Part model, mm, in its own coordinate system. A direction names the side the tool comes from. Coordinates: 2 decimals unless noted, no trailing zeros. Write each loop counter-clockwise with the first axis right and the second up, starting at its lowest first coordinate (ties: lowest second). Pieces come first, ordered by that corner, then holes. Notation, with made-up numbers: (61, 89) -> (67, 89) arc R17 cw to (67, 103) -> close; hole circle Ø5 at (88, -7). An arc over 180 degrees is marked (long way). Write item = value, one per line.
from build123d import *

# Parameters (mm, degrees)
EXTRUDE_1_DEPTH     = 25
SKETCH_2_R          = 1.5
CUT_EXTRUDE_1_DEPTH = 8
SKETCH_3_R          = 1.5
CUT_EXTRUDE_2_DEPTH = 8
CUT_EXTRUDE_3_DEPTH = 8
SKETCH_6_R          = 1.5
CUT_EXTRUDE_4_DEPTH = 94.766234905
FILLET_1_R          = 0.5


with BuildPart() as part:
    # 草图1 → 凸台-拉伸1 (new body)
    with BuildSketch(Plane.XY):
        Polygon((0, 0), (-88, 0), (0, 21.94086425), align=None)
    extrude(amount=EXTRUDE_1_DEPTH)

    # 草图2 → 切除-拉伸1 (cut)
    with BuildSketch(Plane.XZ):
        with Locations(Location((-7.5, 19.5, 0), (0, 0, 270))):
            Circle(SKETCH_2_R)
        with Locations(Location((-7.5, 5.5, 0), (0, 0, 90))):
            Circle(SKETCH_2_R)
    extrude(amount=-CUT_EXTRUDE_1_DEPTH, mode=Mode.SUBTRACT)

    # 草图3 → 切除-拉伸2 (cut)
    with BuildSketch(Plane(origin=(-5.150305914, 20.656748763, 0), x_dir=(0.9702957262759981, 0.24192189559966132, 0), z_dir=(-0.2419218955996613, 0.970295726275998, 0))):
        with Locations(Location((-4.692024529, -5.5, 0), (0, 0, 180))):
            Circle(SKETCH_3_R)
        with Locations(Location((-4.692024529, -19.5, 0), (0, 0, 180))):
            Circle(SKETCH_3_R)
    extrude(amount=-CUT_EXTRUDE_2_DEPTH, mode=Mode.SUBTRACT)

    # 草图5 → 切除-拉伸3 (cut)
    with BuildSketch(Plane.XY.offset(22)):
        Polygon((-77.5, 1.371304016), (-77.5, 2.61794403), (-82.5, 1.371304016), align=None)
    cut_extrude_3 = extrude(amount=-CUT_EXTRUDE_3_DEPTH, mode=Mode.SUBTRACT)

    # 草图6 → 切除-拉伸4 (cut, through all)
    with BuildSketch(Plane(origin=(0, 1.371304016, 0), x_dir=(1, 0, 0), z_dir=(0, 1, 0))):
        with Locations(Location((-80.5, -18, 0), (0, 0, 180))):
            Circle(SKETCH_6_R)
    cut_extrude_4 = extrude(amount=-CUT_EXTRUDE_4_DEPTH, mode=Mode.SUBTRACT)

    # 镜向1: 切除-拉伸3, 切除-拉伸4 across plane
    add(cut_extrude_3.mirror(Plane.XY.offset(12.5)), mode=Mode.SUBTRACT)
    add(cut_extrude_4.mirror(Plane.XY.offset(12.5)), mode=Mode.SUBTRACT)

    # 圆角1
    fillet_1_edges = [part.edges().sort_by_distance(p)[0] for p in [
        (-80, 1.371304016, 14),
        (-77.5, 1.371304016, 18),
        (-77.5, 1.994624023, 14),
        (-80, 1.371304016, 22),
        (-77.5, 1.994624023, 22),
        (-80, 1.371304016, 3),
        (-77.5, 1.994624023, 3),
        (-77.5, 1.371304016, 7),
        (-80, 1.371304016, 11),
        (-77.5, 1.994624023, 11),
    ]]
    fillet(fillet_1_edges, radius=FILLET_1_R)


solid = part.part
Q1. Saw through at C-C on z = 2. Give the cut face in (x, y), and give its area (3 significant figures).
Model answer:
outline = (-88, 0) -> (0, 0) -> (0, 21.94) -> close
area = 965 mm²
Q2. Mould opens along Y. For faces 6 (the face through (-43, 0, 12)), 7 (the face through (-7.59, 15.98, 4.59)), 8 (the face through (-24, 6, 0)) say: released by +Y, released by -Y, zero draft, split by the parting line, or undercut.
Model answer:
face_6 = released by -Y
face_7 = undercut
face_8 = zero draft
Q3. Saw through at D-D on x = -65.5. Give the cut face in (y, z), and give its area (3 significant figures).
Model answer:
outline = (0, 0) -> (5.61, 0) -> (5.61, 25) -> (0, 25) -> close
area = 140 mm²
Q4. Pin check, flat tips, straight feed: pin 1 (3 mm diameter, centred on x = -63.5, z = 20.5, fed in from +Y); pin 2 (0.5 mm diameter, centred on x = -79.5, y = 2.5, fed in from +Z) (3 decimals); pin 3 (1.8 mm diameter, centred on x = -7.5, z = 5.5, fed in from +Y); pin 4 (4 mm diameter, centred on x = -80.5, z = 7, fed in from +Y). Stop position of each tip, or through.
Model answer:
pin_1 = 6.48
pin_2 = through
pin_3 = 20.3
pin_4 = 1.37
Q5. Probe line 1 (Z direction, x = -80.5, y = 0.35); line 2 (X direction, y = 2.5, z = 5.5); line 3 (Z direction, x = -8.5, y = 18.5). List the from-to ranges inside material, lowest first. Write a range as from..to.
Model answer:
line_1 = 0..5.5, 8.5..16.5, 19.5..25
line_2 = -77.5..-9, -6..0
line_3 = 0..4.32, 6.68..18.32, 20.68..25
Q6. Saw through at B-B on x = -7.5. Count the separate pieces of the cut face and the enclosed holes in it, and give its area (3 significant figures).
Model answer:
separate_pieces = 1
enclosed_holes = 2
area = 431 mm²
Q7. Saw through at A-A on y = 6.5. Give the cut face in (x, z), and give its area (3 significant figures).
Model answer:
outline = (-61.93, 0) -> (0, 0) -> (0, 25) -> (-61.93, 25) -> close; hole circle Ø3 at (-7.5, 5.5); hole circle Ø3 at (-7.5, 19.5)
area = 1,530 mm²
Q8. Which spindle directions (+Z, -Z, +X, -X, +Y, -Y) get a long thin tool onto all of the face, cutting with end or side? Do faces 1 (the face through (-24, 6, 25)), 2 (the face through (-8.4, 3.9, 20.7)), 3 (the face through (-78.8, 1.371, 7)), 4 (the face through (-81.886, 0.695, 7.575)), 5 (the face through (-7.747, 11.764, 19.521)). Say none if no direction does.
Model answer:
face_1 = +Z, +X, -X, +Y, -Y
face_2 = -Y
face_3 = -X, +Y
face_4 = +Y, -Y
face_5 = none
